Design review of the part built by this model. Coordinates are the model's own, in mm. Face numbers are marked on the shaded views. Coordinates: 2 decimals unless noted, no trailing zeros. Loops run counter-clockwise (first coordinate to the right, second up) from the corner with the lowest first, then second, coordinate; pieces in that order, holes last. Notation, with made-up numbers: (32.5, 89) -> (38.5, 89) arc R28 ccw to (38.5, 126) -> close; hole circle Ø8 at (40, -11.5). An arc over 180 degrees is marked (long way). One line per item, written item: value. Start each with the question number.
1. Draft analysis for pull direction X (two halves, no side actions). For the marked faces 1, 2 and 3, state which applies: pulls with the +X half, pulls with the -X half, needs draft (parallel to the pull), parting line crosses it, or undercut.
2. Add section C-C on z = -5.5. Write out the cut boundary in (x, y).
3. Add section B-B on x = -10. Write out the cut boundary in (y, z), plus the area to 3 significant figures.
4. For probe 1 along X at (y, z) = (-4.3, 11.5); probe 2 along X at (y, z) = (-1.3, 8) (3 decimals); probe 3 along Z at (x, y) = (12.5, -3.2), list the stretches that pass through material, from the lowest coordinate up.
5. Insertion check: pin 1 (2 mm diameter, centred on y = -1, z = 5, fed in from -X); pin 2 (1 mm diameter, centred on y = -1.5, z = -4, fed in from +X); pin 3 (1 mm diameter, centred on x = -10, y = -2, fed in from +Z). Each pin has a flat end and moves straight along its axis. Give the tip position at first contact, or say it passes through.
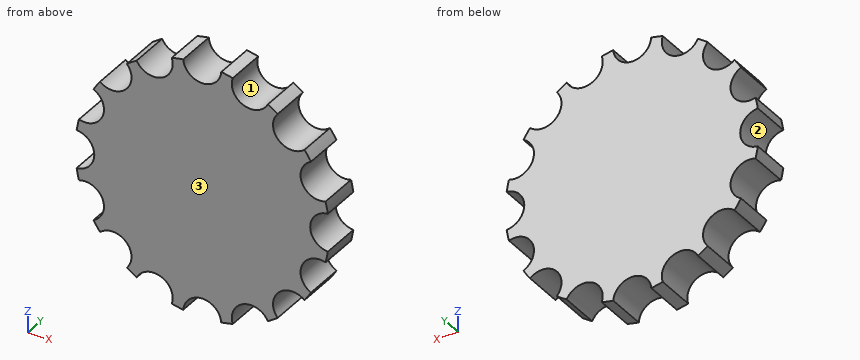
```python
from build123d import *

# Parameters (mm, degrees)
F0_R            = 14
F1_DEPTH        = 4.5
F3_DEPTH        = 4.501
F3_COPIES_COUNT = 16


# Not quite as in the source:
# - a pattern or mirror of a feature is missing from the dataset's text; its kind, count and spacing are read off the source's solid


with BuildPart() as f1:
    # F0 (on Front) → F1 (new body)
    with BuildSketch(Plane.XZ):
        Circle(F0_R)
    extrude(amount=F1_DEPTH)

    # F2 (on face) → F3 (cut, through all)
    with BuildSketch(Plane.XZ.offset(4.5)):
        with BuildLine():
            ThreePointArc((2.0940854209, 13.8425), (0, 14), (-2.0940854209, 13.8425))
            ThreePointArc((-2.0940854209, 13.8425), (0, 11.9), (2.0940854209, 13.8425))
        make_face()
    f3 = extrude(amount=-F3_DEPTH, mode=Mode.SUBTRACT)

    # F3_copies: F3 ×16 about axis
    f3_copies_axis = Axis((0, 0, 0), (0, 1, 0))
    for i in range(1, F3_COPIES_COUNT):
        add(f3.rotate(f3_copies_axis, i * 360 / F3_COPIES_COUNT), mode=Mode.SUBTRACT)


solid = f1.part
```
Worked answers:
1. face 1: undercut
1. face 2: pulls with the -X half
1. face 3: needs draft
2. outline: (-10.84, -4.5) -> (10.84, -4.5) -> (10.84, 0) -> (-10.84, 0) -> close
3. outline: (-4.5, -7.8) -> (0, -7.8) -> (0, 7.8) -> (-4.5, 7.8) -> close
3. area: 70.2 mm²
4. probe 1: x = -7.98 to -6.89, -3.82 to 3.82, 6.89 to 7.98
4. probe 2: x = -11.489 to -10.795, -9.004 to 9.004, 10.795 to 11.489
4. probe 3: z = -3.3 to -1.47, 1.47 to 3.3
5. pin 1: stops at x = -11.33
5. pin 2: stops at x = 11.95
5. pin 3: stops at z = 7.89
